Geometry check sheet. Reference: the model listing, model coordinates, mm. Coordinates: 2 decimals unless noted, no trailing zeros. Loops run counter-clockwise (first coordinate to the right, second up) from the corner with the lowest first, then second, coordinate; pieces in that order, holes last. Notation, with made-up numbers: (89, -14.5) - (148, -14.5) arc R23 cw to (148, 23.5) - close; hole circle Ø6 at (15, -28.75). An arc over 180 degrees is marked (long way). Write each question's results on one line, items separated by ' | '. Start each with the question number.
(1) Sectioned sample at A-A (y = 0). Enter the section's corners in (x, z), plus the area to 3 significant figures.
(2) Go/stop test with flat-tipped pins: pin 1 Ø2 at (y, z) = (-48.5, 3) entering from -X; pin 2 Ø2 at (x, z) = (86.5, 3) entering from +Y; pin 3 Ø1.5 at (x, z) = (-29, 1) entering from -Y. Record where each tip stops, or that it passes through.
(3) Sectioned sample at C-C (y = 18). Enter the section's corners in (x, z), plus the area to 3 significant figures.
(4) Material ranges on probe 1 along Y at (x, z) = (0, 2); probe 2 along Y at (x, z) = (76.2, 1.5); probe 3 along X at (y, z) = (9.5, 3.75), recorded low to high.
(5) Sectioned sample at B-B (x = -76.2). Enter the section's corners in (y, z), plus the area to 3 significant figures.
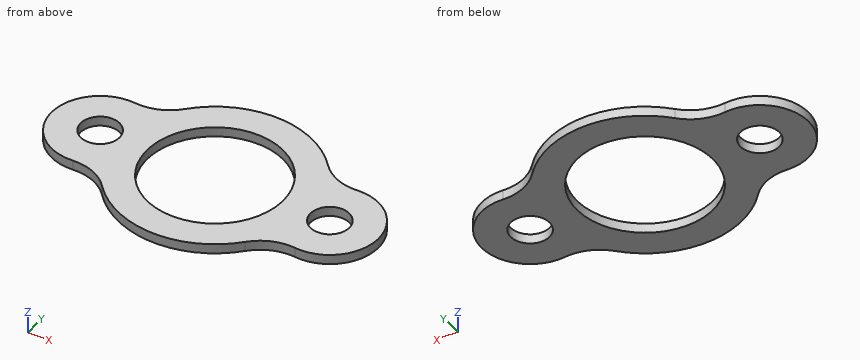
from build123d import *

# Parameters (mm, degrees)
F0_R     = 12.7
F0_R_2   = 44.45
F1_DEPTH = 6.35
F2_R     = 31.75


# Not quite as in the source:
# - a feature names something its author has since deleted; it is built from what else it names


with BuildPart() as f1:
    # F0 (on Top) → F1 (new body)
    with BuildSketch(Plane.XY):
        with BuildLine():
            ThreePointArc((-57.94375, 25.976370723), (-107.95, 0), (-57.94375, -25.976370723))
            ThreePointArc((-57.94375, -25.976370723), (0, -63.5), (57.94375, -25.976370723))
            ThreePointArc((57.94375, -25.976370723), (107.95, 0), (57.94375, 25.976370723))
            ThreePointArc((57.94375, 25.976370723), (0, 63.5), (-57.94375, 25.976370723))
        make_face()
        with Locations((-76.2, 0)):
            Circle(F0_R, mode=Mode.SUBTRACT)
        Circle(F0_R_2, mode=Mode.SUBTRACT)
        with Locations((76.2, 0)):
            Circle(F0_R, mode=Mode.SUBTRACT)
    extrude(amount=F1_DEPTH)

    # F2
    f2_edges = [f1.edges().sort_by_distance(p)[0] for p in [
        (-57.94375, -25.976371, 3.175),
        (57.94375, -25.976371, 3.175),
        (-57.94375, 25.976371, 3.175),
        (57.94375, 25.976371, 3.175),
    ]]
    fillet(f2_edges, radius=F2_R)


solid = f1.part
Outcome:
1) outline: (-107.95, 0) - (-88.9, 0) - (-88.9, 6.35) - (-107.95, 6.35) - close; (-63.5, 0) - (-44.45, 0) - (-44.45, 6.35) - (-63.5, 6.35) - close; (44.45, 0) - (63.5, 0) - (63.5, 6.35) - (44.45, 6.35) - close; (88.9, 0) - (107.95, 0) - (107.95, 6.35) - (88.9, 6.35) - close | area: 484 mm2
2) pin 1: stops at x = -42.14 | pin 2: stops at y = 30.36 | pin 3: stops at y = -56.87
3) outline: (-102.35, 0) - (-40.64, 0) - (-40.64, 6.35) - (-102.35, 6.35) - close; (40.64, 0) - (102.35, 0) - (102.35, 6.35) - (40.64, 6.35) - close | area: 784 mm2
4) probe 1: y = -63.5 to -44.45, 44.45 to 63.5 | probe 2: y = -31.75 to -12.7, 12.7 to 31.75 | probe 3: x = -106.5 to -84.63, -67.77 to -43.42, 43.42 to 67.77, 84.63 to 106.5
5) outline: (-31.75, 0) - (-12.7, 0) - (-12.7, 6.35) - (-31.75, 6.35) - close; (12.7, 0) - (31.75, 0) - (31.75, 6.35) - (12.7, 6.35) - close | area: 242 mm2
